Input: dimensioned drawing with shaded views. Units: mm. Origin: part minimum x, y, z. A direction names the side the tool comes from. Coordinates: 2 decimals unless noted, no trailing zeros. Loops run counter-clockwise (first coordinate to the right, second up) from the corner with the lowest first, then second, coordinate; pieces in that order, holes last. Notation, with made-up numbers: (-6.5, 72) - (8.5, 72) arc R32 ccw to (8.5, 107) - close; hole circle Ø6 at (25, 17.5). An arc over 180 degrees is marked (long way). Put each result on its own line as item: value. Start each with the question number.
1) Reachability of the marked faces 1, 2 and 3 from +Z, -Z, +X, -X, +Y, -Y: full face, straight path, thin tool, end or side. Return the list, or none.
2) Section A-A on x = 60. Output: boundary loops of the cut face in (y, z), and give its area (3 significant figures).
3) Contact query for flat-ended pins moving along their axis: pin 1 Ø2 at (y, z) = (45.5, 11) entering from +X; pin 2 Ø1.5 at (x, z) = (16.5, 19) entering from +Y; pin 3 Ø12 at (y, z) = (59.5, 22.5) entering from -X. Output: stop coordinate, or through.
4) Section B-B on z = 15. Output: boundary loops of the cut face in (x, y).
5) Section D-D on y = 61. Output: boundary loops of the cut face in (x, z).
6) Draft query along X for the marked faces 4, 5 and 6. Return one class per face: +X half, -X half, draft (parallel to the pull), parting line (faces both ways), or undercut.
7) Section C-C on z = 2.5. Output: boundary loops of the cut face in (x, y), and give its area (3 significant figures).
8) Material intervals for line 1 along X through (y, z) = (68.75, 15); line 2 along Z through (x, y) = (60, 65); line 3 along Z through (x, y) = (60, 66.25), sorted ascending. Write a range as from..to.
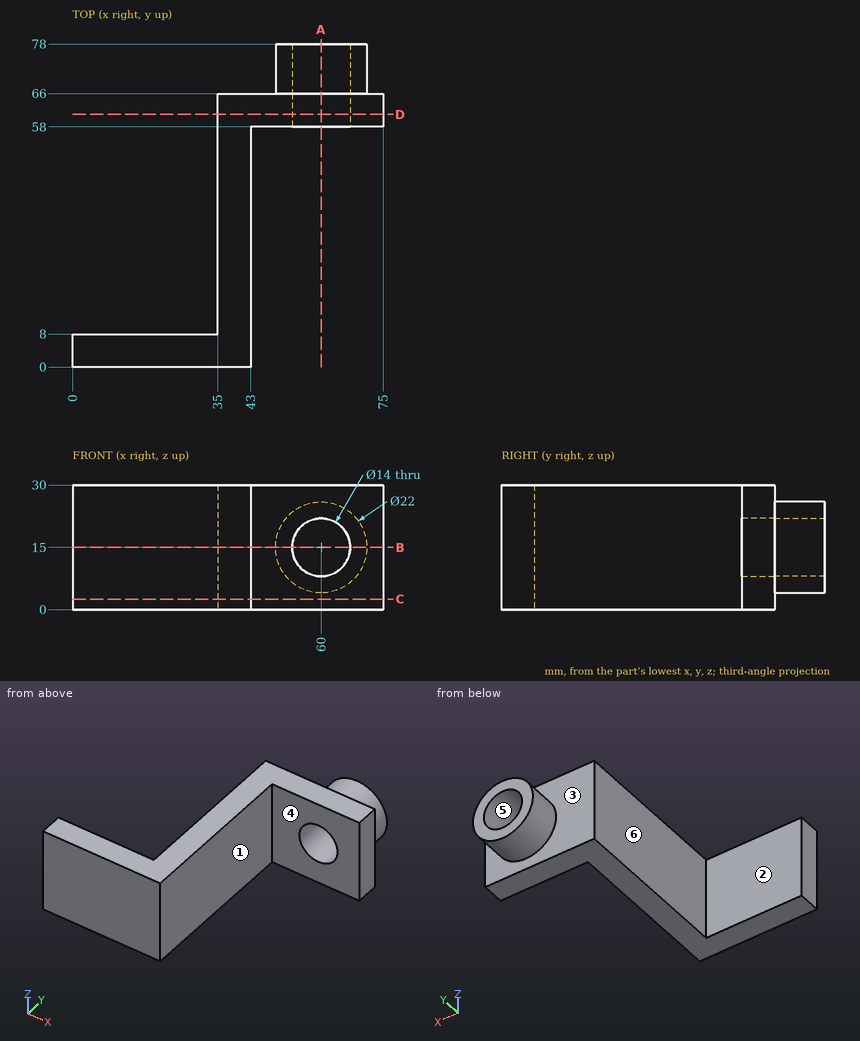
Answer block:
1. face 1: +Z, -Z, +X, -Y
1. face 2: +Z, -Z, -X, +Y
1. face 3: +Y
2. outline: (58, 0) - (66, 0) - (66, 4) - (78, 4) - (78, 8) - (58, 8) - close; (58, 22) - (78, 22) - (78, 26) - (66, 26) - (66, 30) - (58, 30) - close
2. area: 224 mm²
3. pin 1: stops at x = 43
3. pin 2: stops at y = 8
3. pin 3: stops at x = 35
4. outline: (0, 0) - (43, 0) - (43, 58) - (53, 58) - (53, 78) - (49, 78) - (49, 66) - (35, 66) - (35, 8) - (0, 8) - close; (67, 58) - (75, 58) - (75, 66) - (71, 66) - (71, 78) - (67, 78) - close
5. outline: (35, 0) - (75, 0) - (75, 30) - (35, 30) - close; hole circle Ø14 at (60, 15)
6. face 4: draft
6. face 5: undercut
6. face 6: -X half
7. outline: (0, 0) - (43, 0) - (43, 58) - (75, 58) - (75, 66) - (35, 66) - (35, 8) - (0, 8) - close
7. area: 1,060 mm²
8. line 1: x = 49..53, 67..71
8. line 2: z = 0..8, 22..30
8. line 3: z = 4..8, 22..26
